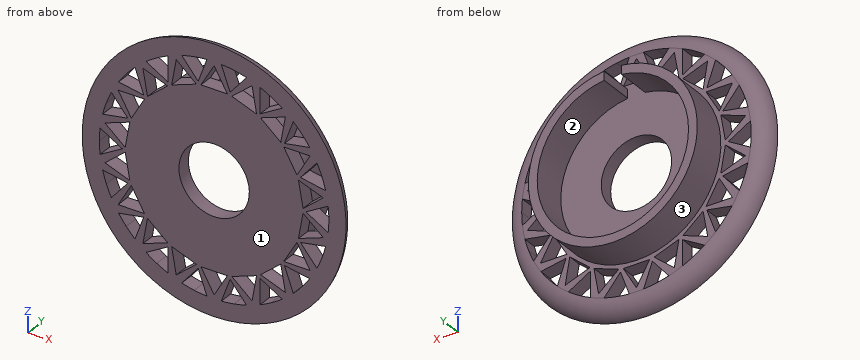
from build123d import *

# Parameters (mm, degrees)
SKETCH1_R           = 75
BOSS_EXTRUDE1_DEPTH = 8
SKETCH2_R           = 48
SKETCH2_R_2         = 43
BOSS_EXTRUDE3_DEPTH = 20
CUT_EXTRUDE2_START  = -20
CUT_EXTRUDE2_DEPTH  = 20
FILLET1_R           = 10
CUT_EXTRUDE3_DEPTH  = 108.935165725
CIRPATTERN1_COUNT   = 18
SKETCH9_R           = 20
CUT_EXTRUDE4_DEPTH  = 108.935165725


with BuildPart() as part:
    # Sketch1 → Boss-Extrude1 (new body)
    with BuildSketch(Plane(origin=(0, 0, 0), x_dir=(1, 0, 0), z_dir=(0, 1, 0))):
        with Locations(Location((0, 0, 0), (0, 0, 270))):
            Circle(SKETCH1_R)
    extrude(amount=BOSS_EXTRUDE1_DEPTH)

    # Sketch2 → Boss-Extrude3 (add)
    with BuildSketch(Plane(origin=(0, 8, 0), x_dir=(1, 0, 0), z_dir=(0, 1, 0))):
        with Locations(Location((0, 0, 0), (0, 0, 270))):
            Circle(SKETCH2_R)
        with Locations(Location((0, 0, 0), (0, 0, 270))):
            Circle(SKETCH2_R_2, mode=Mode.SUBTRACT)
    extrude(amount=BOSS_EXTRUDE3_DEPTH)

    # Sketch7 → Cut-Extrude2 (cut)
    with BuildSketch(Plane(origin=(0, 28, 0), x_dir=(1, 0, 0), z_dir=(0, 1, 0)).offset(CUT_EXTRUDE2_START)):
        with BuildLine():
            Line((0, -43), (-5, -43))
            Line((-5, -43), (-5, -47.738873049))
            ThreePointArc((-5, -47.738873049), (-2.503407043, -47.934673809), (0, -48))
            ThreePointArc((0, -48), (2.503407043, -47.934673809), (5, -47.738873049))
            Line((5, -47.738873049), (5, -43))
            Line((5, -43), (0, -43))
        make_face()
        with BuildLine():
            ThreePointArc((0, -48), (-2.503407043, -47.934673809), (-5, -47.738873049))
            Line((-5, -47.738873049), (-5, -48))
            Line((-5, -48), (0, -48))
        make_face()
        with BuildLine():
            ThreePointArc((5, -47.738873049), (2.503407043, -47.934673809), (0, -48))
            Line((0, -48), (5, -48))
            Line((5, -48), (5, -47.738873049))
        make_face()
        with BuildLine():
            ThreePointArc((4.966536902, -42.712217353), (2.4874338, -42.927994049), (0, -43))
            Line((0, -43), (5, -43))
            Line((5, -43), (4.966536902, -42.712217353))
        make_face()
        with BuildLine():
            Line((-4.966536902, -42.712217353), (-5, -43))
            Line((-5, -43), (0, -43))
            ThreePointArc((0, -43), (-2.4874338, -42.927994049), (-4.966536902, -42.712217353))
        make_face()
    extrude(amount=CUT_EXTRUDE2_DEPTH, mode=Mode.SUBTRACT)

    # Fillet1
    # the kernel refuses this fillet: 10 mm, written as the material it takes off along each edge
    with BuildSketch(Plane(origin=(0, 8, 0), x_dir=(0, 0, 1), z_dir=(-1, 0, 0))) as fillet1_piece_1:
        with BuildLine():
            CenterArc((65.202041029, -10), FILLET1_R, 11.536959033, 78.463040967)
            Line((65.202041029, 0), (65.202041029, 0.2))
            Line((65.202041029, 0.2), (75, 0.2))
            Line((75, 0.2), (75.2, 0))
            ThreePointArc((75.2, 0), (75.2, -4), (75.195959179, -7.96))
            Line((75.195959179, -7.96), (75, -8))
        make_face()
    revolve(axis=Axis((0, 8, 0), (0, 1, 0)), mode=Mode.SUBTRACT)

    # Sketch8 → Cut-Extrude3 (cut, through all)
    with BuildSketch(Plane(origin=(0, 8, 0), x_dir=(1, 0, 0), z_dir=(0, 1, 0))):
        with BuildLine():
            Line((-64.795971013, -7.265555367), (-52.211659972, 0))
            Line((-52.211659972, 0), (-64.795971013, 7.265555367))
            ThreePointArc((-64.795971013, 7.265555367), (-65.100444372, 3.638447047), (-65.202041029, 0))
            ThreePointArc((-65.202041029, 0), (-65.100444372, -3.638447047), (-64.795971013, -7.265555367))
        make_face()
        Polygon((-50.542748983, 1.296350736), (-47.938026318, 16.068467031), (-62.03341563, 10.938164881), align=None)
    cut_extrude3 = extrude(amount=-CUT_EXTRUDE3_DEPTH, mode=Mode.SUBTRACT)

    # CirPattern1: Cut-Extrude3 ×18 about axis
    cirpattern1_axis = Axis((0, 0, 0), (0, 1, 0))
    for i in range(1, CIRPATTERN1_COUNT):
        add(cut_extrude3.rotate(cirpattern1_axis, i * 360 / CIRPATTERN1_COUNT), mode=Mode.SUBTRACT)

    # Sketch9 → Cut-Extrude4 (cut, through all)
    with BuildSketch(Plane(origin=(0, 8, 0), x_dir=(1, 0, 0), z_dir=(0, 1, 0))):
        with Locations(Location((0, 0, 0), (0, 0, 270))):
            Circle(SKETCH9_R)
    extrude(amount=-CUT_EXTRUDE4_DEPTH, mode=Mode.SUBTRACT)


solid = part.part
Can you work these out from the model? Positions are in its coordinate system, mm. Face numbers are marked on the shaded views. Coordinates: 2 decimals unless noted, no trailing zeros. Loops run counter-clockwise (first coordinate to the right, second up) from the corner with the lowest first, then second, coordinate; pieces in that order, holes last. Notation, with made-up numbers: M -15,28 L 7,28 A9 cw 7,45 Z; hole C 33.5,-11.5 d9. An arc over 180 degrees is marked long. Answer as CSV lines item,"result". Start each with the question number.
1. Suppose I cut it at A-A, the plane y = 10.5. List the corners of the cut face in (x, z) for me, plus the area to 3 significant figures.
2. Suppose I cut it at B-B, the plane z = 13.5. Count the separate pieces of the cut face and the enclosed holes in it, plus the area to 3 significant figures.
3. Thinking about a two-plate mould opening in X: for the marked faces 1, 2 and 3, which applies, +X half, -X half, draft (parallel to the pull), parting line (faces both ways), or undercut?
4. For pin 1 Ø6.5 at (y, z) = (5.5, 50.5) entering from -X; pin 2 Ø9 at (x, y) = (43.5, 5) entering from +Z; pin 3 Ø4 at (y, z) = (6, 55.5) entering from +X, each with a flat end and sliding along its axis, tell me the tip position at first contact or that it passes through.
5. If I drill on probe 1 along Z at (x, y) = (-33, 5); probe 2 along X at (y, z) = (17.25, 0); probe 3 along X at (y, z) = (6.5, -21), over which ranges is the centre line in solid material (lowest first)? Write a range as [from, to].
Output:
1,outline,"M -5,43 L -5,47.74 A48 ccw long 5,47.74 L 5,43 L 4.97,42.71 A43 cw long -4.97,42.71 Z"
1,area,"1,380 mm^2"
2,separate pieces,"4"
2,enclosed holes,"0"
2,area,"1,010 mm^2"
3,face 1,"draft"
3,face 2,"undercut"
3,face 3,"parting line"
4,pin 1,"stops at x = -55.81"
4,pin 2,"stops at z = 62.6"
4,pin 3,"stops at x = 48.63"
5,probe 1,"z = [-64.38, -56.23], [-49.2, -45.53], [-37.58, 37.58], [45.53, 49.2], [56.23, 64.38]"
5,probe 2,"x = [-48, -43], [43, 48]"
5,probe 3,"x = [-67.27, -61.73], [-51.7, -48.49], [-45.61, 45.61], [48.49, 51.7], [61.73, 67.27]"
